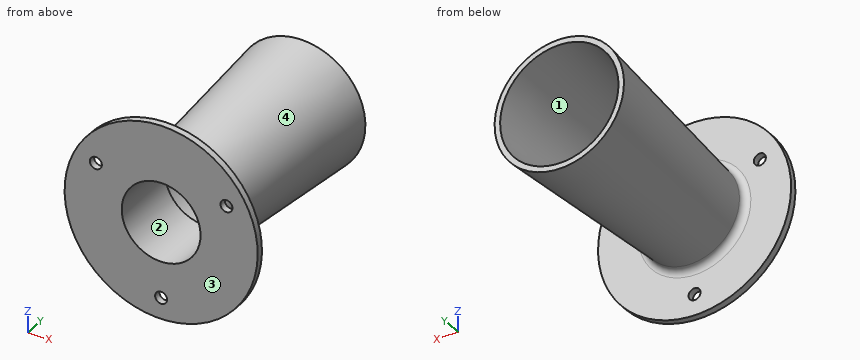
from build123d import *

# Parameters (mm, degrees)
FILLET1_R          = 2
SKETCH2_R          = 1.75
CUT_EXTRUDE1_DEPTH = 3


with BuildPart() as part:
    # Sketch1 → Revolve1 (revolve)
    with BuildSketch(Plane.XY, mode=Mode.PRIVATE) as revolve1_sk:
        Polygon((11.5, 0), (11.5, 20.222386647), (14, 20.222386647), (17.273009701, 65.222386647), (18.877236254, 65.222386647), (14.278847703, 2), (28.171211947, 2), (28.171211947, 0), align=None)
    revolve(revolve1_sk.sketch.rotate(Axis((0, 70.073472281, 0), (0, -1, 0)), 90), axis=Axis((0, 70.073472281, 0), (0, -1, 0)))  # turned: the seam where the file's is

    # Fillet1
    fillet1_edges = [part.edges().sort_by_distance(p)[0] for p in [
        (0, 2, -14.278847703),
    ]]
    fillet(fillet1_edges, radius=FILLET1_R)

    # Sketch2 → Cut-Extrude1 (cut, through all)
    with BuildSketch(Plane(origin=(0, 2, 0), x_dir=(1, 0, 0), z_dir=(0, 1, 0))):
        with Locations(Location((0, 22, 0), (0, 0, 270))):  # turned: the seam where the file's is
            Circle(SKETCH2_R)
        with Locations(Location((19.052558883, -11, 0), (0, 0, 270))):  # turned: the seam where the file's is
            Circle(SKETCH2_R)
        with Locations(Location((-19.052558883, -11, 0), (0, 0, 270))):  # turned: the seam where the file's is
            Circle(SKETCH2_R)
    extrude(amount=-CUT_EXTRUDE1_DEPTH, mode=Mode.SUBTRACT)


solid = part.part
Verification items for the finished model (mm, model axes). Face numbers are marked on the shaded views. Give positions to 0.01 mm unless a question says otherwise; leave off trailing zeros. Loops run counter-clockwise (first coordinate to the right, second up) from the corner with the lowest first, then second, coordinate; pieces in that order, holes last.
1) Draft check along Y on the marked faces 1, 2, 3 and 4. Enter one of: pulls with the +Y half, pulls with the -Y half, needs draft (parallel to the pull), parting line crosses it, or undercut.
2) Sectioned sample at A-A, the plane z = -22. Enter the section's corners in (x, y).
3) Depth check by flat-ended pin: pin 1 Ø5.5 at (x, z) = (-19.05, 11) entering from +Y; pin 2 Ø5 at (x, y) = (-8.5, 49.5) entering from +Z; pin 3 Ø8 at (y, z) = (48.5, 4.5) entering from -X. Enter the tip coordinate at first touch or a pass-through.
4) Sectioned sample at D-D, the plane z = 24.5. Enter the section's corners in (x, y).
5) Thickness scan on line 1 along Z through (x, y) = (11, 46); line 2 along Y through (x, z) = (21.5, -7); line 3 along Z through (x, y) = (2, 19). Record the ranges inside material, lowest first.
6) Sectioned sample at C-C, the plane y = 34.5. Enter the section's corners in (x, z), then the cut area to 3 significant figures.
7) Sectioned sample at B-B, the plane x = 0. Enter the section's corners in (y, z).
Answers:
1. face 1: pulls with the +Y half
1. face 2: needs draft
1. face 3: pulls with the -Y half
1. face 4: undercut
2. outline: (-17.6, 0) - (-1.75, 0) - (-1.75, 2) - (-17.6, 2) - close; (1.75, 0) - (17.6, 0) - (17.6, 2) - (1.75, 2) - close
3. pin 1: stops at y = 2
3. pin 2: stops at z = 16.71
3. pin 3: stops at x = -17.79
4. outline: (-13.91, 0) - (13.91, 0) - (13.91, 2) - (-13.91, 2) - close
5. line 1: z = -13.58 to -11.45, 11.45 to 13.58
5. line 2: y = 0 to 2
5. line 3: z = -15.39 to -11.32, 11.32 to 15.39
6. outline: circle Ø33.29 at (0, 0); hole circle Ø30.08 at (0, 0)
6. area: 160 mm2
7. outline: (0, -28.17) - (2, -28.17) - (2, -23.75) - (0, -23.75) - close; (0, -20.25) - (2, -20.25) - (2, -16.43) arc R2 cw to (4.15, -14.43) - (65.22, -18.88) - (65.22, -17.27) - (20.22, -14) - (20.22, -11.5) - (0, -11.5) - close; (0, 11.5) - (20.22, 11.5) - (20.22, 14) - (65.22, 17.27) - (65.22, 18.88) - (4.15, 14.43) arc R2 cw to (2, 16.43) - (2, 28.17) - (0, 28.17) - close
